The listing builds one solid part. Answer for the finished solid, in the listing's coordinates (mm). Round coordinates to 2 decimals unless told otherwise and drop trailing zeros. Order: outer loops, then holes, each group sorted by start corner. A loop starts at its lowest first (then second) coordinate and runs counter-clockwise, first axis right, second up. Notation, with made-up numbers: (15, 30.25) -> (61, 30.25) arc R28 cw to (61, 67.25) -> close; hole circle Ø9 at (73.25, 9.5). An arc over 180 degrees is marked (long way). Answer in a Markdown table with one row per item. Add a question column.
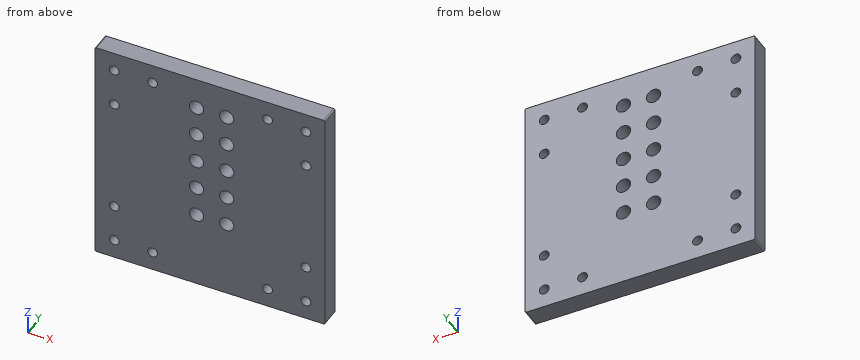
```python
from build123d import *

# Parameters (mm, degrees)
SKETCH1_W           = 152.4
SKETCH1_H           = 152.4
SKETCH1_R           = 4.75
BOSS_EXTRUDE1_DEPTH = 12.7
FILLET1_R           = 1
SKETCH11_R          = 3.2639
CUT_EXTRUDE1_DEPTH  = 12.7
SKETCH12_R          = 4.75
CUT_EXTRUDE2_DEPTH  = 12.7


with BuildPart() as part:
    # Sketch1 → Boss-Extrude1 (new body)
    # profile 1 of 13: a face of its own
    with BuildSketch(Plane(origin=(0, 0, 0), x_dir=(1, 0, 0), z_dir=(0, 1, 0))):
        with Locations((76.2, -76.2)):
            Rectangle(SKETCH1_W, SKETCH1_H)
        with Locations((12.7, -38.1)):
            Circle(SKETCH1_R, mode=Mode.SUBTRACT)
        with Locations((12.7, -114.3)):
            Circle(SKETCH1_R, mode=Mode.SUBTRACT)
        with Locations((38.1, -139.7)):
            Circle(SKETCH1_R, mode=Mode.SUBTRACT)
        with Locations((114.3, -139.7)):
            Circle(SKETCH1_R, mode=Mode.SUBTRACT)
        with Locations((139.7, -114.3)):
            Circle(SKETCH1_R, mode=Mode.SUBTRACT)
        with Locations((139.7, -38.1)):
            Circle(SKETCH1_R, mode=Mode.SUBTRACT)
        with Locations((114.3, -12.7)):
            Circle(SKETCH1_R, mode=Mode.SUBTRACT)
        with Locations((38.1, -12.7)):
            Circle(SKETCH1_R, mode=Mode.SUBTRACT)
        with Locations((12.7, -139.7)):
            Circle(SKETCH1_R, mode=Mode.SUBTRACT)
        with Locations((139.7, -139.7)):
            Circle(SKETCH1_R, mode=Mode.SUBTRACT)
        with Locations((139.7, -12.7)):
            Circle(SKETCH1_R, mode=Mode.SUBTRACT)
        with Locations((12.7, -12.7)):
            Circle(SKETCH1_R, mode=Mode.SUBTRACT)
    # profile 2 of 13: a face of its own
    with BuildSketch(Plane(origin=(0, 0, 0), x_dir=(1, 0, 0), z_dir=(0, 1, 0))):
        with Locations((12.7, -12.7)):
            Circle(SKETCH1_R)
    # profile 3 of 13: a face of its own
    with BuildSketch(Plane(origin=(0, 0, 0), x_dir=(1, 0, 0), z_dir=(0, 1, 0))):
        with Locations((139.7, -12.7)):
            Circle(SKETCH1_R)
    # profile 4 of 13: a face of its own
    with BuildSketch(Plane(origin=(0, 0, 0), x_dir=(1, 0, 0), z_dir=(0, 1, 0))):
        with Locations((139.7, -139.7)):
            Circle(SKETCH1_R)
    # profile 5 of 13: a face of its own
    with BuildSketch(Plane(origin=(0, 0, 0), x_dir=(1, 0, 0), z_dir=(0, 1, 0))):
        with Locations((12.7, -139.7)):
            Circle(SKETCH1_R)
    # profile 6 of 13: a face of its own
    with BuildSketch(Plane(origin=(0, 0, 0), x_dir=(1, 0, 0), z_dir=(0, 1, 0))):
        with Locations((38.1, -12.7)):
            Circle(SKETCH1_R)
    # profile 7 of 13: a face of its own
    with BuildSketch(Plane(origin=(0, 0, 0), x_dir=(1, 0, 0), z_dir=(0, 1, 0))):
        with Locations((12.7, -38.1)):
            Circle(SKETCH1_R)
    # profile 8 of 13: a face of its own
    with BuildSketch(Plane(origin=(0, 0, 0), x_dir=(1, 0, 0), z_dir=(0, 1, 0))):
        with Locations((139.7, -38.1)):
            Circle(SKETCH1_R)
    # profile 9 of 13: a face of its own
    with BuildSketch(Plane(origin=(0, 0, 0), x_dir=(1, 0, 0), z_dir=(0, 1, 0))):
        with Locations((114.3, -12.7)):
            Circle(SKETCH1_R)
    # profile 10 of 13: a face of its own
    with BuildSketch(Plane(origin=(0, 0, 0), x_dir=(1, 0, 0), z_dir=(0, 1, 0))):
        with Locations((139.7, -114.3)):
            Circle(SKETCH1_R)
    # profile 11 of 13: a face of its own
    with BuildSketch(Plane(origin=(0, 0, 0), x_dir=(1, 0, 0), z_dir=(0, 1, 0))):
        with Locations((114.3, -139.7)):
            Circle(SKETCH1_R)
    # profile 12 of 13: a face of its own
    with BuildSketch(Plane(origin=(0, 0, 0), x_dir=(1, 0, 0), z_dir=(0, 1, 0))):
        with Locations((12.7, -114.3)):
            Circle(SKETCH1_R)
    # profile 13 of 13: a face of its own
    with BuildSketch(Plane(origin=(0, 0, 0), x_dir=(1, 0, 0), z_dir=(0, 1, 0))):
        with Locations((38.1, -139.7)):
            Circle(SKETCH1_R)
    extrude(amount=BOSS_EXTRUDE1_DEPTH)

    # Fillet1
    fillet1_edges = [part.edges().sort_by_distance(p)[0] for p in [
        (152.4, 6.35, 152.4),
        (0, 6.35, 152.4),
        (0, 6.35, 0),
        (152.4, 6.35, 0),
    ]]
    fillet(fillet1_edges, radius=FILLET1_R)

    # Sketch11 → Cut-Extrude1 (cut)
    with BuildSketch(Plane(origin=(0, 12.7, 0), x_dir=(1, 0, 0), z_dir=(0, 1, 0))):
        with Locations(Location((38.1, -12.7, 0), (0, 0, 270))):
            Circle(SKETCH11_R)
        with Locations(Location((12.7, -12.7, 0), (0, 0, 270))):
            Circle(SKETCH11_R)
        with Locations(Location((139.7, -12.7, 0), (0, 0, 270))):
            Circle(SKETCH11_R)
        with Locations(Location((12.7, -38.1, 0), (0, 0, 270))):
            Circle(SKETCH11_R)
        with Locations(Location((114.3, -12.7, 0), (0, 0, 270))):
            Circle(SKETCH11_R)
        with Locations(Location((139.7, -38.1, 0), (0, 0, 270))):
            Circle(SKETCH11_R)
        with Locations(Location((139.7, -114.3, 0), (0, 0, 270))):
            Circle(SKETCH11_R)
        with Locations(Location((114.3, -139.7, 0), (0, 0, 270))):
            Circle(SKETCH11_R)
        with Locations(Location((12.7, -114.3, 0), (0, 0, 270))):
            Circle(SKETCH11_R)
        with Locations(Location((38.1, -139.7, 0), (0, 0, 270))):
            Circle(SKETCH11_R)
        with Locations(Location((139.7, -139.7, 0), (0, 0, 270))):
            Circle(SKETCH11_R)
        with Locations(Location((12.7, -139.7, 0), (0, 0, 270))):
            Circle(SKETCH11_R)
    extrude(amount=-CUT_EXTRUDE1_DEPTH, mode=Mode.SUBTRACT)

    # Sketch12 → Cut-Extrude2 (cut)
    with BuildSketch(Plane.XZ):
        with Locations(Location((67.2, 131.495, 0), (0, 0, 270))):
            Circle(SKETCH12_R)
        with Locations(Location((87.2, 131.495, 0), (0, 0, 270))):
            Circle(SKETCH12_R)
        with Locations(Location((87.2, 111.495, 0), (0, 0, 270))):
            Circle(SKETCH12_R)
        with Locations(Location((67.2, 111.495, 0), (0, 0, 270))):
            Circle(SKETCH12_R)
        with Locations(Location((67.2, 91.495, 0), (0, 0, 270))):
            Circle(SKETCH12_R)
        with Locations(Location((67.2, 71.495, 0), (0, 0, 270))):
            Circle(SKETCH12_R)
        with Locations(Location((67.2, 51.495, 0), (0, 0, 270))):
            Circle(SKETCH12_R)
        with Locations(Location((87.2, 51.495, 0), (0, 0, 270))):
            Circle(SKETCH12_R)
        with Locations(Location((87.2, 71.495, 0), (0, 0, 270))):
            Circle(SKETCH12_R)
        with Locations(Location((87.2, 91.495, 0), (0, 0, 270))):
            Circle(SKETCH12_R)
    extrude(amount=-CUT_EXTRUDE2_DEPTH, mode=Mode.SUBTRACT)


solid = part.part
```
1. This flat-tipped pin is pushed along its axis until it touches: pin 1 (4 mm diameter, centred on x = 38.1, z = 139.7, fed in from -Y). Where does it stop, or does it pass through?
2. The part is cut by section C-C (x = 38.1). Give the vertices of the cut face in (y, z), then the cut area to 3 significant figures.
3. The part is cut by section D-D (x = 12.7). Give the vertices of the cut face in (y, z).
4. The part is cut by section A-A (z = 139.7). Give the vertices of the cut face in (x, y), then the cut area to 3 significant figures.
5. The part is cut by section B-B (y = 5.5). Give the number of separate pieces and of enclosed holes in the cut face, then the cut area to 3 significant figures.
6. Straight lines are drawn through the part: line 1 along X through (y, z) = (4.5, 12.7); line 2 along Z through (x, y) = (13, 5). For each, find the intervals that lie inside material, in ascending order.
Report:
| question | item | result |
|---|---|---|
| 1 | pin 1 | passes through |
| 2 | outline | (0, 0) -> (12.7, 0) -> (12.7, 9.44) -> (0, 9.44) -> close; (0, 15.96) -> (12.7, 15.96) -> (12.7, 136.44) -> (0, 136.44) -> close; (0, 142.96) -> (12.7, 142.96) -> (12.7, 152.4) -> (0, 152.4) -> close |
| 2 | area | 1,770 mm^2 |
| 3 | outline | (0, 0) -> (12.7, 0) -> (12.7, 9.44) -> (0, 9.44) -> close; (0, 15.96) -> (12.7, 15.96) -> (12.7, 34.84) -> (0, 34.84) -> close; (0, 41.36) -> (12.7, 41.36) -> (12.7, 111.04) -> (0, 111.04) -> close; (0, 117.56) -> (12.7, 117.56) -> (12.7, 136.44) -> (0, 136.44) -> close; (0, 142.96) -> (12.7, 142.96) -> (12.7, 152.4) -> (0, 152.4) -> close |
| 4 | outline | (0, 0) -> (9.44, 0) -> (9.44, 12.7) -> (0, 12.7) -> close; (15.96, 0) -> (34.84, 0) -> (34.84, 12.7) -> (15.96, 12.7) -> close; (41.36, 0) -> (111.04, 0) -> (111.04, 12.7) -> (41.36, 12.7) -> close; (117.56, 0) -> (136.44, 0) -> (136.44, 12.7) -> (117.56, 12.7) -> close; (142.96, 0) -> (152.4, 0) -> (152.4, 12.7) -> (142.96, 12.7) -> close |
| 4 | area | 1,600 mm^2 |
| 5 | separate pieces | 1 |
| 5 | enclosed holes | 22 |
| 5 | area | 22,100 mm^2 |
| 6 | line 1 | x = 0 to 9.44, 15.96 to 34.84, 41.36 to 111.04, 117.56 to 136.44, 142.96 to 152.4 |
| 6 | line 2 | z = 0 to 9.45, 15.95 to 34.85, 41.35 to 111.05, 117.55 to 136.45, 142.95 to 152.4 |
